Part model, mm, in its own coordinate system. Face numbers are marked on the shaded views. A direction names the side the tool comes from. Give positions to 0.01 mm unless a question says otherwise; leave off trailing zeros. Write each loop counter-clockwise with the first axis right and the second up, starting at its lowest first coordinate (ties: lowest second). Pieces come first, ordered by that corner, then holes.
```python
from build123d import *

# Parameters (mm, degrees)
SKETCH3_R           = 6
SKETCH3_R_2         = 1.5
BOSS_EXTRUDE1_DEPTH = 16
FILLET1_R           = 3
SKETCH4_R           = 1.5
CUT_EXTRUDE1_DEPTH  = 41.620192023


with BuildPart() as part:
    # Sketch3 → Boss-Extrude1 (new body)
    # profile 1 of 5: a face of its own
    with BuildSketch(Plane(origin=(0, 0, 0), x_dir=(1, 0, 0), z_dir=(0, 1, 0))):
        with BuildLine():
            Line((14, 12), (14, 6))
            Line((14, 6), (20, 6))
            ThreePointArc((20, 6), (15.757359313, 7.757359313), (14, 12))
        make_face()
    # profile 2 of 5: a face of its own
    with BuildSketch(Plane(origin=(0, 0, 0), x_dir=(1, 0, 0), z_dir=(0, 1, 0))):
        with Locations((20, 12)):
            Circle(SKETCH3_R)
        with Locations(Location((20, 12, 0), (0, 0, 270))):
            Circle(SKETCH3_R_2, mode=Mode.SUBTRACT)
    # profile 3 of 5: a face of its own
    with BuildSketch(Plane(origin=(0, 0, 0), x_dir=(1, 0, 0), z_dir=(0, 1, 0))):
        with BuildLine():
            Line((14, 6), (0, 6))
            ThreePointArc((0, 6), (4.242640687, 4.242640687), (6, 0))
            ThreePointArc((6, 0), (4.242640687, -4.242640687), (0, -6))
            Line((0, -6), (26, -6))
            Line((26, -6), (26, 5))
            Line((26, 5), (26, 12))
            ThreePointArc((26, 12), (24.242640687, 7.757359313), (20, 6))
            Line((20, 6), (14, 6))
        make_face()
    # profile 4 of 5: a face of its own
    with BuildSketch(Plane(origin=(0, 0, 0), x_dir=(1, 0, 0), z_dir=(0, 1, 0))):
        Circle(SKETCH3_R)
        with Locations(Location((0, 0, 0), (0, 0, 270))):
            Circle(SKETCH3_R_2, mode=Mode.SUBTRACT)
    # profile 5 of 5: a face of its own
    with BuildSketch(Plane(origin=(0, 0, 0), x_dir=(1, 0, 0), z_dir=(0, 1, 0))):
        Polygon((26, 5), (26, -6), (26.875327872, -6), (35, -6), (35, 5), align=None)
    extrude(amount=BOSS_EXTRUDE1_DEPTH)

    # Fillet1
    fillet1_edges = [part.edges().sort_by_distance(p)[0] for p in [
        (14, 8, -6),
    ]]
    fillet(fillet1_edges, radius=FILLET1_R)

    # Sketch4 → Cut-Extrude1 (cut, through all)
    with BuildSketch(Plane(origin=(0, 0, -5), x_dir=(-1, 0, 0), z_dir=(0, 0, -1))):
        with Locations((-30.5, 12)):
            Circle(SKETCH4_R)
        with Locations((-30.5, 4)):
            Circle(SKETCH4_R)
    extrude(amount=-CUT_EXTRUDE1_DEPTH, mode=Mode.SUBTRACT)


solid = part.part
```
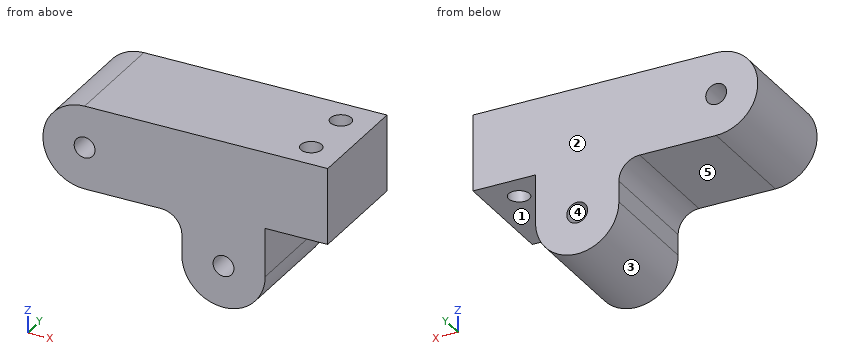
1) 3-axis set-ups, long thin cutter, end or side, ignore diameter. For the marked faces 1 and 2: which of +Z, -Z, +X, -X, +Y, -Y reach the whole face in a straight line?
Answers follow:
face 1: -Z, +X, +Y, -Y
face 2: +Z, -Z, +X, -X, +Y
2) Two-plate mould, pull along X, no slides. Class the marked faces 3, 4 and 5: +X half, -X half, draft (parallel to the pull), parting line (faces both ways), or undercut.
Answers follow:
face 3: parting line
face 4: undercut
face 5: draft
3) Saw through at B-B, the plane x = 20. Write the cut outline in (y, z), then the cut area to 3 significant figures.
Answers follow:
outline: (0, -18) - (16, -18) - (16, -13.5) - (0, -13.5) - close; (0, -10.5) - (16, -10.5) - (16, 6) - (0, 6) - close
area: 336 mm2
4) Saw through at D-D, the plane z = 2.75. Write the cut outline in (x, y).
Answers follow:
outline: (-5.33, 0) - (35, 0) - (35, 16) - (-5.33, 16) - close; hole circle Ø3 at (30.5, 4); hole circle Ø3 at (30.5, 12)
5) Pin check, flat tips, straight feed: pin 1 Ø6 at (x, y) = (12.5, 12.5) entering from -Z; pin 2 Ø3.5 at (x, y) = (4.5, 6) entering from -Z; pin 3 Ø5 at (y, z) = (9.5, -13.5) entering from -X; pin 4 Ø3 at (x, z) = (1.5, -8.5) entering from +Y. Stop position of each tip, or through.
Answers follow:
pin 1: stops at z = -15.97
pin 2: stops at z = -6
pin 3: stops at x = 14
pin 4: passes through
6) Saw through at A-A, the plane y = 4. Write the cut outline in (x, z).
Answers follow:
outline: (0, -6) - (11, -6) arc R3 cw to (14, -9) - (14, -12) arc R6 ccw to (26, -12) - (26, -5) - (29, -5) - (29, 6) - (0, 6) arc R6 ccw to start; (32, -5) - (35, -5) - (35, 6) - (32, 6) - close; hole circle Ø3 at (0, 0); hole circle Ø3 at (20, -12)
7) Wall check: L1, parallel to Y at x = 30.5, z = -2; L2, parallel to X at y = 4.5, z = -12; L3, parallel to X at y = 7.5, z = 0. Give the ranges that are in metal, low to high.
Answers follow:
L1: y = 0 to 2.5, 5.5 to 10.5, 13.5 to 16
L2: x = 14 to 18.5, 21.5 to 26
L3: x = -6 to -1.5, 1.5 to 35
8) Saw through at C-C, the plane y = 14. Write the cut outline in (x, z), then the cut area to 3 significant figures.
Answers follow:
outline: (0, -6) - (11, -6) arc R3 cw to (14, -9) - (14, -12) arc R6 ccw to (26, -12) - (26, -5) - (35, -5) - (35, 6) - (0, 6) arc R6 ccw to start; hole circle Ø3 at (0, 0); hole circle Ø3 at (20, -12)
area: 584 mm2
